Autodesk Inventor part; units mm, degrees
ref_plane "YZ Plane" through (0, 0, 0) normal (1, 0, 0) x (0, 1, 0)
ref_plane "XZ Plane" through (0, 0, 0) normal (0, 1, 0) x (-1, 0, 0)
ref_plane "XY Plane" through (0, 0, 0) normal (0, 0, 1) x (1, 0, 0)
sketch "Sketch1" plane through (0, 0, 0) normal (0, 0, 1) x (1, 0, 0)
  line L0 (-20, 0) -> (20, 0)
  line L1 (20, 0) -> (20, -50)
  line L2 (20, -50) -> (-20, -50)
  line L3 (-20, -50) -> (-20, 0)
  line L4 (-35, -80) -> (35, -80)
  line L5 (35, -80) -> (35, -50)
  line L6 (35, -50) -> (-35, -50)
  line L7 (-35, -50) -> (-35, -80)
  circle A0 centre (-15, -65) radius 2.5
  circle A1 centre (15, -65) radius 2.5
  line L8 (0, -80) -> (0, -50) construction
  circle A2 centre (-30, -55) radius 2.5
  circle A3 centre (30, -55) radius 2.5
  circle A4 centre (30, -75) radius 2.5
  circle A5 centre (-30, -75) radius 2.5
  line L9 (-35, -65) -> (35, -65) construction
  point P0 (0, 0)
  point P1 (0, 0)
  dimension "d0" = 40
  dimension "d1" = 50
  dimension "d33" = 70
  dimension "d34" = 5
  dimension "d35" = 30
  dimension "d36" = 30
  dimension "d38" = 5
  dimension "d39" = 5
extrude "Plate1" add sketch "Sketch1" along normal blind 2
fillet "Corner Round1" radius 2 8 edges at (-20, -50, 1) (-35, -50, 1) (20, -50, 1) (35, -50, 1) (35, -80, 1) (-35, -80, 1) (-20, 0, 1) (20, 0, 1)
equation "\"d2\" = Thickness"
equation "\"BendReliefWidth\" = Thickness"
equation "\"BendReliefDepth\" = 0.5 * Thickness"
equation "\"CornerReliefSize\" = 4 * Thickness"
equation "\"MinimumRemnant\" = 2 * Thickness"
equation "\"TransitionRadius\" = BendRadius"
equation "\"JacobiRadiusSize\" = BendRadius"
equation "\"GapSize\" = Thickness"
properties part number "NDM 11.030 plate" material "Stainless Steel"
Model file for the job. Use its own axes, mm. A direction names the side the tool comes from. Give positions to 0.01 mm unless a question says otherwise; leave off trailing zeros. Loops run counter-clockwise (first coordinate to the right, second up) from the corner with the lowest first, then second, coordinate; pieces in that order, holes last.
Item 1: Drill centre lines: line 1 along Y through (x, z) = (-30, 1.5); line 2 along X through (y, z) = (-66, 1.25); line 3 along X through (y, z) = (-54, 0.35). Where is each one in solid material? Low to high.
Check values:
line 1: y = -80 to -77.5, -72.5 to -57.5, -52.5 to -50
line 2: x = -35 to -17.29, -12.71 to 12.71, 17.29 to 35
line 3: x = -35 to -32.29, -27.71 to 27.71, 32.29 to 35
Item 2: Drop flat-ended pins along their axis: P1, Ø12, axis at x = 15, y = -33, coming from the -Z side; P2, Ø0.6, axis at x = -27, z = 1, coming from the +Y side; P3, Ø0.6, axis at y = -33.5, z = 1, coming from the +X side; P4, Ø1, axis at y = -30.5, z = 1.5, coming from the -X side. Give the stop position or say it passes through.
Check values:
P1: stops at z = 0
P2: stops at y = -50
P3: stops at x = 20
P4: stops at x = -20
Item 3: Which spindle directions (+Z, -Z, +X, -X, +Y, -Y) get a long thin tool onto all of the face, cutting with end or side? Do faces 1 (the face through (20, -25, 1)), 2 (the face through (-32.5, -55.1, 1)). Say none if no direction does.
Check values:
face 1: +Z, -Z, +X, +Y
face 2: +Z, -Z
Item 4: Slice it at C-C (z = 0.65). Write the cut outline in (x, y).
Check values:
outline: (-35, -78) arc R2 ccw to (-33, -80) - (33, -80) arc R2 ccw to (35, -78) - (35, -52) arc R2 ccw to (33, -50) - (22, -50) arc R2 cw to (20, -48) - (20, -2) arc R2 ccw to (18, 0) - (-18, 0) arc R2 ccw to (-20, -2) - (-20, -48) arc R2 cw to (-22, -50) - (-33, -50) arc R2 ccw to (-35, -52) - close; hole circle Ø5 at (-30, -75); hole circle Ø5 at (-30, -55); hole circle Ø5 at (-15, -65); hole circle Ø5 at (15, -65); hole circle Ø5 at (30, -75); hole circle Ø5 at (30, -55)
Item 5: Slice it at D-D (x = 15). Write the cut outline in (y, z).
Check values:
outline: (-80, 0) - (-67.5, 0) - (-67.5, 2) - (-80, 2) - close; (-62.5, 0) - (0, 0) - (0, 2) - (-62.5, 2) - close
Item 6: Slice it at A-A (x = 30). Write the cut outline in (y, z), plus the area to 3 significant figures.
Check values:
outline: (-80, 0) - (-77.5, 0) - (-77.5, 2) - (-80, 2) - close; (-72.5, 0) - (-57.5, 0) - (-57.5, 2) - (-72.5, 2) - close; (-52.5, 0) - (-50, 0) - (-50, 2) - (-52.5, 2) - close
area: 40.0 mm2
Item 7: Slice it at B-B (y = -75). Write the cut outline in (x, z), plus the area to 3 significant figures.
Check values:
outline: (-35, 0) - (-32.5, 0) - (-32.5, 2) - (-35, 2) - close; (-27.5, 0) - (27.5, 0) - (27.5, 2) - (-27.5, 2) - close; (32.5, 0) - (35, 0) - (35, 2) - (32.5, 2) - close
area: 120 mm2
Item 8: Mould opens along X. For faces 3 (the face through (28.16, -56.69, 0.99)), 4 (the face through (28, -50, 1)), 5 (the face through (34.43, -50.6, 1.01)) say: +X half, -X half, draft (parallel to the pull), parting line (faces both ways), or undercut.
Check values:
face 3: undercut
face 4: draft
face 5: +X half
